Can you work these out from the model? Positions are in its coordinate system, mm. A direction names the side the tool comes from. Round coordinates to 2 decimals unless told otherwise and drop trailing zeros. Order: outer loops, then holes, each group sorted by start corner. A loop starts at its lowest first (then second) coordinate and runs counter-clockwise, first axis right, second up. Notation, with made-up numbers: (72.25, 23) -> (126.25, 23) arc R3 cw to (126.25, 27) -> close; hole circle Ø5 at (6.5, -31). An arc over 180 degrees is marked (long way). One line per item, written item: value.
```python
from build123d import *

# Parameters (mm, degrees)
F0_R     = 50.8
F0_R_2   = 5.1562
F0_W     = 19.05
F0_H     = 19.05
F1_DEPTH = 12.7
F2_R     = 25.4
F3_DEPTH = 3.048


with BuildPart() as f1:
    # F0 (on Front) → F1 (new body)
    with BuildSketch(Plane.XZ):
        Circle(F0_R)
        with Locations((0, -41.275)):
            Circle(F0_R_2, mode=Mode.SUBTRACT)
        with Locations((-41.275, 0)):
            Circle(F0_R_2, mode=Mode.SUBTRACT)
        Rectangle(F0_W, F0_H, mode=Mode.SUBTRACT)
        with Locations((41.275, 0)):
            Circle(F0_R_2, mode=Mode.SUBTRACT)
        with Locations((0, 41.275)):
            Circle(F0_R_2, mode=Mode.SUBTRACT)
    extrude(amount=F1_DEPTH)

    # F2 (on Front) → F3 (cut)
    with BuildSketch(Plane.XZ):
        Circle(F2_R)
    extrude(amount=F3_DEPTH, mode=Mode.SUBTRACT)


solid = f1.part
```
Q1. Will these pins go through, and if not, where does the flat tip stop? pin 1 Ø7.5 at (x, y) = (4, -9.5) entering from +Z; pin 2 Ø2 at (x, y) = (-7.5, -8.5) entering from +Z; pin 3 Ø3 at (y, z) = (-1.5, -21.5) entering from +X; pin 4 Ø3 at (y, z) = (-10, -1.5) entering from -X.
Answers below:
pin 1: z = 50.8
pin 2: z = 50.38
pin 3: x = 46.7
pin 4: x = -50.8
Q2. I want a section at A-A on x = 0. List the corners of the cut face in (y, z) for me (3 decimals).
Answers below:
outline: (-12.7, -50.8) -> (0, -50.8) -> (0, -46.431) -> (-12.7, -46.431) -> close; (-12.7, -36.119) -> (0, -36.119) -> (0, -25.4) -> (-3.048, -25.4) -> (-3.048, -9.525) -> (-12.7, -9.525) -> close; (-12.7, 9.525) -> (-3.048, 9.525) -> (-3.048, 25.4) -> (0, 25.4) -> (0, 36.119) -> (-12.7, 36.119) -> close; (-12.7, 46.431) -> (0, 46.431) -> (0, 50.8) -> (-12.7, 50.8) -> close
Q3. Please list where these lines run through material, in increasing order: line 1 along Z through (x, y) = (0, -4.5) (3 decimals); line 2 along X through (y, z) = (-0.5, -4); line 3 along Z through (x, y) = (8.5, -2).
Answers below:
line 1: -50.8 to -46.431, -36.119 to -9.525, 9.525 to 36.119, 46.431 to 50.8
line 2: -50.64 to -44.53, -38.02 to -25.08, 25.08 to 38.02, 44.53 to 50.64
line 3: -50.08 to -23.94, 23.94 to 50.08
Q4. We'd pull the mould along Z, two halves only. Please class faces 1 (the face through (11, -12.7, 1)), 2 (the face through (-11.012, -6.261, -49.592)), 3 (the face through (37.183, -6.261, -3.137)), 4 (the face through (0, -8, 9.525)): released by +Z, released by -Z, zero draft, split by the parting line, or undercut.
Answers below:
face 1: zero draft
face 2: split by the parting line
face 3: undercut
face 4: undercut
Q5. I want a section at D-D on y = -5. List the corners of the cut face in (x, z) for me (3 decimals).
Answers below:
outline: circle Ø101.6 at (0, 0); hole circle Ø10.312 at (-41.275, 0); hole (-9.525, -9.525) -> (9.525, -9.525) -> (9.525, 9.525) -> (-9.525, 9.525) -> close; hole circle Ø10.312 at (0, -41.275); hole circle Ø10.312 at (0, 41.275); hole circle Ø10.312 at (41.275, 0)
Q6. I want a section at C-C on x = -44. List the corners of the cut face in (y, z) for me, plus the area to 3 significant figures.
Answers below:
outline: (-12.7, -25.39) -> (0, -25.39) -> (0, -4.38) -> (-12.7, -4.38) -> close; (-12.7, 4.38) -> (0, 4.38) -> (0, 25.39) -> (-12.7, 25.39) -> close
area: 534 mm^2
Q7. On a 3-axis mill with a long thin cutter (end or side, diameter ignored), from which of +Z, -Z, +X, -X, +Y, -Y can I reach the whole of each face in a straight line? I mean faces 5 (the face through (-5.506, -1.503, -24.796)), 6 (the face through (-9.525, -8, 0)), 7 (the face through (-23.3, 0, -10.6)). Say none if no direction works.
Answers below:
face 5: +Y
face 6: +Y, -Y
face 7: +Z, -Z, +X, -X, +Y
Q8. I want a section at B-B on z = 0. List the corners of the cut face in (x, y) for me (3 decimals).
Answers below:
outline: (-50.8, -12.7) -> (-46.431, -12.7) -> (-46.431, 0) -> (-50.8, 0) -> close; (-36.119, -12.7) -> (-9.525, -12.7) -> (-9.525, -3.048) -> (-25.4, -3.048) -> (-25.4, 0) -> (-36.119, 0) -> close; (9.525, -12.7) -> (36.119, -12.7) -> (36.119, 0) -> (25.4, 0) -> (25.4, -3.048) -> (9.525, -3.048) -> close; (46.431, -12.7) -> (50.8, -12.7) -> (50.8, 0) -> (46.431, 0) -> close
